Verification items for the finished model (mm, model axes). A direction names the side the tool comes from. Give positions to 0.01 mm unless a question says otherwise; leave off trailing zeros. Loops run counter-clockwise (first coordinate to the right, second up) from the corner with the lowest first, then second, coordinate; pieces in that order, holes last. Notation, with made-up numbers: M 89,25 L 148,25 A20 ccw 148,35 Z; hole C 17.5,-32 d7. An arc over 180 degrees is marked long. Put each result on its own line as item: value. Start each with the question number.
from build123d import *

# Parameters (mm, degrees)
EXTRUDE_1_DEPTH     = 20
FILLET_2_R          = 2
FILLET_4_R          = 2
SKETCH_2_R          = 6.8
CUT_EXTRUDE_2_DEPTH = 20


with BuildPart() as part:
    # 草图1 → 凸台-拉伸1 (new body)
    with BuildSketch(Plane.XY):
        Polygon((-27.351383791, 53.289188169), (-27.351383791, -8.710811831), (-25.351383791, -8.710811831), (-25.351383791, 51.289188169), (14.948616209, 51.289188169), (14.948616209, -8.710811831), (17.423079102, -8.710811831), (16.948616209, 53.289188169), align=None)
    extrude(amount=EXTRUDE_1_DEPTH)

    # 圆角2
    fillet_2_edges = [part.edges().sort_by_distance(p)[0] for p in [
        (-27.351383791, 53.289188169, 10),
    ]]
    fillet(fillet_2_edges, radius=FILLET_2_R)

    # 圆角4
    fillet_4_edges = [part.edges().sort_by_distance(p)[0] for p in [
        (16.948616209, 53.289188169, 10),
    ]]
    fillet(fillet_4_edges, radius=FILLET_4_R)

    # 草图2 → 切除-拉伸2 (cut)
    with BuildSketch(Plane(origin=(0, 53.289188169, 0), x_dir=(1, 0, 0), z_dir=(0, 1, 0))):
        with Locations(Location((-5.193760445, -10, 0), (0, 0, 180))):
            Circle(SKETCH_2_R)
    extrude(amount=-CUT_EXTRUDE_2_DEPTH, mode=Mode.SUBTRACT)


solid = part.part
Q1. Cross-section at B-B, the plane x = -6.5. Record the boundary of the cut face in (y, z), then the cut area to 3 significant figures.
Q2. Go/stop test with flat-tipped pins: pin 1 (6 mm diameter, centred on x = -5.5, z = 15, fed in from -Y); pin 2 (1 mm diameter, centred on y = 41, z = 14.5, fed in from +X). Record where each tip stops, or that it passes through.
Q3. Cross-section at D-D, the plane y = 27.5. Record the boundary of the cut face in (x, z), then the cut area to 3 significant figures.
Q4. Release check for a two-part mould opening along X. For faces 1 (the face through (-25.351, 21, 10)), 2 (the face through (-26.78, 52.69, 10.14)), 3 (the face through (16, 53, 10)) record: pulls with the +X half, pulls with the -X half, needs draft (parallel to the pull), parting line crosses it, or undercut.
Q5. Cross-section at A-A, the plane z = 10. Record the boundary of the cut face in (x, y), then the cut area to 3 significant figures.
Q6. Cross-section at C-C, the plane z = 17.75. Record the boundary of the cut face in (x, y).
Q7. Scan lines: L1, parallel to Y at x = -11, z = 14.25; L2, parallel to X at y = 1, z = 13.25; L3, parallel to X at y = 30.5, z = 8.5. Record each from-to range of solid material in increasing order.
Q8. Set-up check for faces 4 (the face through (-26, -8.711, 10)), 5 (the face through (14.949, 22, 10)): record each of +Z, -Z, +X, -X, +Y, -Y from which the full face is reachable in a straight line by a thin tool's end or side.
Ans:
1. outline: M 51.29,0 L 53.29,0 L 53.29,3.33 L 51.29,3.33 Z; M 51.29,16.67 L 53.29,16.67 L 53.29,20 L 51.29,20 Z
1. area: 13.3 mm^2
2. pin 1: stops at y = 51.29
2. pin 2: stops at x = 17.05
3. outline: M -27.35,0 L -25.35,0 L -25.35,20 L -27.35,20 Z; M 14.95,0 L 17.15,0 L 17.15,20 L 14.95,20 Z
3. area: 83.9 mm^2
4. face 1: undercut
4. face 2: pulls with the -X half
4. face 3: pulls with the +X half
5. outline: M -27.35,-8.71 L -25.35,-8.71 L -25.35,51.29 L -11.99,51.29 L -11.99,53.29 L -25.35,53.29 A2 ccw -27.35,51.29 Z; M 1.61,51.29 L 14.95,51.29 L 14.95,-8.71 L 17.42,-8.71 L 16.96,51.3 A2 ccw 14.96,53.29 L 1.61,53.29 Z
5. area: 314 mm^2
6. outline: M -27.35,-8.71 L -25.35,-8.71 L -25.35,51.29 L 14.95,51.29 L 14.95,-8.71 L 17.42,-8.71 L 16.96,51.3 A2 ccw 14.96,53.29 L -25.35,53.29 A2 ccw -27.35,51.29 Z
7. L1: y = 51.29 to 53.29
7. L2: x = -27.35 to -25.35, 14.95 to 17.35
7. L3: x = -27.35 to -25.35, 14.95 to 17.12
8. face 4: +Z, -Z, +X, -X, -Y
8. face 5: +Z, -Z, -Y
